Model file for the job. Use its own axes, mm. A direction names the side the tool comes from. Coordinates: 2 decimals unless noted, no trailing zeros. Order: outer loops, then holes, each group sorted by start corner. A loop starts at its lowest first (then second) coordinate and runs counter-clockwise, first axis right, second up. Notation, with made-up numbers: M -7.75,23 L 47.25,23 A33 cw 47.25,60 Z; hole C 74,53.25 d7. An arc over 180 degrees is marked long. Return JSON: item names as keys, results as strings.
```python
from build123d import *

# Parameters (mm, degrees)
SKETCH1_W           = 96
SKETCH1_H           = 55
BOSS_EXTRUDE1_DEPTH = 1.5
FILLET1_R           = 8


with BuildPart() as part:
    # Sketch1 → Boss-Extrude1 (new, symmetric)
    with BuildSketch(Plane.XY):
        Rectangle(SKETCH1_W, SKETCH1_H)
        with BuildLine():
            Line((-5, -16.1), (-5, -5.5))
            ThreePointArc((-5, -5.5), (0, -0.5), (5, -5.5))
            Line((5, -5.5), (5, -16.1))
            ThreePointArc((5, -16.1), (0, -21.1), (-5, -16.1))
        make_face(mode=Mode.SUBTRACT)
    extrude(amount=BOSS_EXTRUDE1_DEPTH, both=True)

    # Fillet1
    fillet1_edges = [part.edges().sort_by_distance(p)[0] for p in [
        (-48, 27.5, 0),
        (48, 27.5, 0),
    ]]
    fillet(fillet1_edges, radius=FILLET1_R)


solid = part.part
```
Item 1: 3-axis set-ups, long thin cutter, end or side, ignore diameter. For faces 1 (the flat face through (-1, -27.5, 0)), 2 (the flat face through (5, -11, 0)): which of +Z, -Z, +X, -X, +Y, -Y reach the whole face in a straight line?
Check result:
{"face 1": "+Z, -Z, +X, -X, -Y", "face 2": "+Z, -Z"}
Item 2: Pull direction X, two halves, no side cores. Call faces 3 (the flat face through (48, -4, 0)), 4 (the cylindrical face through (0.1, -21.1, 0)), 5 (the flat face through (-1, 0, -1.5)): +X half, -X half, draft (parallel to the pull), parting line (faces both ways), or undercut.
Check result:
{"face 3": "+X half", "face 4": "undercut", "face 5": "draft"}
Item 3: Saw through at C-C (x = 0). Write the cut outline in (y, z), and give its area (3 significant figures).
Check result:
{"outline": "M -27.5,-1.5 L -21.1,-1.5 L -21.1,1.5 L -27.5,1.5 Z; M -0.5,-1.5 L 27.5,-1.5 L 27.5,1.5 L -0.5,1.5 Z", "area": "103 mm2"}
Item 4: Wall check: line 1 (X direction, y = -9, z = 0.6); line 2 (X direction, y = -3.5, z = -0.15); line 3 (X direction, y = 25, z = 1.45). Give the ranges that are in metal, low to high.
Check result:
{"line 1": "x = -48 to -5, 5 to 48", "line 2": "x = -48 to -4.58, 4.58 to 48", "line 3": "x = -45.81 to 45.81"}
Item 5: Saw through at B-B (z = 0.8). Write the cut outline in (x, y), and give its area (3 significant figures).
Check result:
{"outline": "M -48,-27.5 L 48,-27.5 L 48,19.5 A8 ccw 40,27.5 L -40,27.5 A8 ccw -48,19.5 Z; hole M -5,-16.1 A5 ccw 5,-16.1 L 5,-5.5 A5 ccw -5,-5.5 Z", "area": "5,070 mm2"}
Item 6: Saw through at A-A (y = -15). Write the cut outline in (x, z), and give its area (3 significant figures).
Check result:
{"outline": "M -48,-1.5 L -5,-1.5 L -5,1.5 L -48,1.5 Z; M 5,-1.5 L 48,-1.5 L 48,1.5 L 5,1.5 Z", "area": "258 mm2"}
